from build123d import *

# Parameters (mm, degrees)
FILLET1_R = 0.5


with BuildPart() as part:
    # Sketch2 → Revolve1 (revolve)
    with BuildSketch(Plane.XY.offset(-3.5), mode=Mode.PRIVATE) as revolve1_sk:
        with BuildLine():
            ThreePointArc((-20.891294302, 94.7), (-21.391294302, 95.2), (-21.891294302, 94.7))
            Line((-21.891294302, 94.7), (-22.675639033, 94.7))
            Line((-22.675639033, 94.7), (-22.675639033, 96.7375))
            Line((-22.675639033, 96.7375), (-21.555, 96.7375))
            Line((-21.555, 96.7375), (-21.555, 103.8368))
            Line((-21.555, 103.8368), (-20.055, 103.8368))
            Line((-20.055, 103.8368), (-20.055, 96.2))
            Line((-20.055, 96.2), (-19.391294302, 95.536294302))
            Line((-19.391294302, 95.536294302), (-19.391294302, 92.5))
            ThreePointArc((-19.391294302, 92.5), (-20.141294302, 92.25), (-20.891294302, 92.5))
            Line((-20.891294302, 92.5), (-20.891294302, 94.7))
        make_face()
    revolve(revolve1_sk.sketch.rotate(Axis((-26, 90.5, -3.5), (0, 1, 0)), 90), axis=Axis((-26, 90.5, -3.5), (0, 1, 0)))

    # Fillet1
    fillet1_edges = [part.edges().sort_by_distance(p)[0] for p in [
        (-26, 103.8368, 0.945),
        (-26, 103.8368, 2.445),
    ]]
    fillet(fillet1_edges, radius=FILLET1_R)


solid = part.part
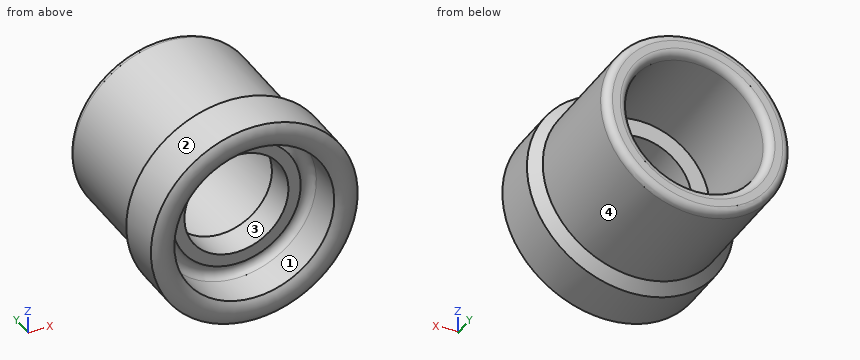
Can you work these out from the model? Positions are in its coordinate system, mm. Face numbers are marked on the shaded views. A direction names the side the tool comes from. Coordinates: 2 decimals unless noted, no trailing zeros. Order: outer loops, then holes, each group sorted by start corner. A loop starts at its lowest first (then second) coordinate and runs counter-clockwise, first axis right, second up. Notation, with made-up numbers: (18, 85.25) - (55, 85.25) arc R13 ccw to (55, 97.25) - close; hole circle Ø4 at (4.5, 14.25). An arc over 180 degrees is marked (long way). Answer as a JSON object with one key per item and string values. Group by question number.
Q1. Imagine slicing it at D-D (y = 97.75). Please give me the cut outline in (x, z) (3 decimals), and give its area (3 significant figures).
Q2. On a 3-axis mill with a long thin cutter (end or side, diameter ignored), from which of +Z, -Z, +X, -X, +Y, -Y can I reach the whole of each face in a straight line? I mean the marked faces 3 and 4. Say none if no direction works.
Q3. We'd pull the mould along X, two halves only. Please class the marked faces 1 and 2: +X half, -X half, draft (parallel to the pull), parting line (faces both ways), or undercut.
Q4. Imagine slicing it at C-C (y = 94). Please give me the cut outline in (x, z).
Q5. I need wall thicknesses on line 1 (Z direction, x = -26, y = 93.65); line 2 (Z direction, x = -26, y = 96.3) (3 decimals); line 3 (X direction, y = 101.75, z = -3.5) (3 decimals). Which ranges of each line are inside material? Lowest first, please. Write a range as from..to.
Q6. Will these pins go through, and if not, where does the flat tip stop? P1, Ø1.5, axis at x = -29.5, y = 100, coming from the +Z side; P2, Ø6, axis at x = -31, y = 101.5, coming from the -Z side; P3, Ø3, axis at x = -29.5, y = 97.5, coming from the +Z side.
Determined:
{
 "1": {"outline": "circle Ø11.89 at (-26, -3.5); hole circle Ø8.89 at (-26, -3.5)", "area": "49.0 mm2"},
 "2": {"face 3": "+Y, -Y", "face 4": "+Y"},
 "3": {"face 1": "undercut", "face 2": "parting line"},
 "4": {"outline": "circle Ø13.22 at (-26, -3.5); hole circle Ø10.22 at (-26, -3.5)"},
 "5": {"line 1": "z = -10.11..-8.61, 1.61..3.11", "line 2": "z = -9.445..-6.824, -0.176..2.445", "line 3": "x = -31.945..-30.445, -21.555..-20.055"},
 "6": {"P1": "stops at z = 1.77", "P2": "stops at z = -9.1", "P3": "stops at z = 2.1"}
}
